from build123d import *

# Parameters (mm, degrees)
SKETCH1_W           = 30
SKETCH1_H           = 34
SKETCH1_R           = 1.625
BOSS_EXTRUDE1_DEPTH = 6
BOSS_EXTRUDE3_START = -6
SKETCH2_R           = 10
SKETCH2_R_2         = 4.05
BOSS_EXTRUDE3_DEPTH = 6
SKETCH3_R           = 2.1
BOSS_EXTRUDE4_DEPTH = 21.376405408
CUT_EXTRUDE1_START  = -10
CUT_EXTRUDE1_DEPTH  = 10
SKETCH5_W           = 4.7
SKETCH5_H           = 23.2
BOSS_EXTRUDE5_DEPTH = 17.376405408
CUT_EXTRUDE2_DEPTH  = 10
SKETCH8_R           = 2.05
CUT_EXTRUDE3_DEPTH  = 10
SKETCH9_W           = 30
SKETCH9_H           = 53.05
SKETCH9_R           = 4.05
BOSS_EXTRUDE6_DEPTH = 6
SKETCH10_R          = 2.05
CUT_EXTRUDE7_DEPTH  = 10
FILLET2_R           = 3.6
FILLET3_R           = 3.6
CHAMFER1_SIZE       = 1
CHAMFER2_SIZE       = 1


with BuildPart() as part:
    # Sketch1 → Boss-Extrude1 (new body)
    with BuildSketch(Plane.XY):
        Rectangle(SKETCH1_W, SKETCH1_H)
        with Locations((-9, 12)):
            Circle(SKETCH1_R, mode=Mode.SUBTRACT)
        with Locations((9, 12)):
            Circle(SKETCH1_R, mode=Mode.SUBTRACT)
        with Locations((-9, -12)):
            Circle(SKETCH1_R, mode=Mode.SUBTRACT)
        with Locations((9, -12)):
            Circle(SKETCH1_R, mode=Mode.SUBTRACT)
    extrude(amount=-BOSS_EXTRUDE1_DEPTH)

    # Sketch2 → Boss-Extrude3 (add)
    with BuildSketch(Plane.XY.offset(BOSS_EXTRUDE3_START)):
        Polygon((-15, -17), (15, -17), (15, -64.6), (-15, -64.6), (-27.6, -64.6), (-27.6, -41.4), (-15, -41.4), align=None)
        with Locations((0, -29)):
            Circle(SKETCH2_R, mode=Mode.SUBTRACT)
        with Locations((0, -54)):
            Circle(SKETCH2_R_2, mode=Mode.SUBTRACT)
    extrude(amount=BOSS_EXTRUDE3_DEPTH)

    # Sketch3 → Boss-Extrude4 (add)
    with BuildSketch(Plane(origin=(0, 0, -6), x_dir=(-1, 0, 0), z_dir=(0, 0, -1))):
        with BuildLine():
            Line((27.6, -61), (27.6, -45))
            ThreePointArc((27.6, -45), (26.545584412, -42.454415588), (24, -41.4))
            Line((24, -41.4), (19.7, -41.4))
            Line((19.7, -41.4), (19.7, -64.6))
            Line((19.7, -64.6), (24, -64.6))
            ThreePointArc((24, -64.6), (26.545584412, -63.545584412), (27.6, -61))
        make_face()
        with Locations(Location((24, -61, 0), (0, 0, 180))):
            Circle(SKETCH3_R, mode=Mode.SUBTRACT)
        with Locations(Location((24, -45, 0), (0, 0, 180))):
            Circle(SKETCH3_R, mode=Mode.SUBTRACT)
    extrude(amount=BOSS_EXTRUDE4_DEPTH)

    # Sketch4 → Cut-Extrude1 (cut)
    with BuildSketch(Plane(origin=(0, 0, -6), x_dir=(-1, 0, 0), z_dir=(0, 0, -1)).offset(CUT_EXTRUDE1_START)):
        with BuildLine():
            ThreePointArc((27.6, -61), (26.545584412, -63.545584412), (24, -64.6))
            Line((24, -64.6), (27.6, -64.6))
            Line((27.6, -64.6), (27.6, -61))
        make_face()
        with BuildLine():
            ThreePointArc((24, -41.4), (26.545584412, -42.454415588), (27.6, -45))
            Line((27.6, -45), (27.6, -41.4))
            Line((27.6, -41.4), (24, -41.4))
        make_face()
    extrude(amount=CUT_EXTRUDE1_DEPTH, mode=Mode.SUBTRACT)

    # Sketch5 → Boss-Extrude5 (add)
    with BuildSketch(Plane(origin=(0, 0, -6), x_dir=(-1, 0, 0), z_dir=(0, 0, -1))):
        with Locations((17.35, -53)):
            Rectangle(SKETCH5_W, SKETCH5_H)
    extrude(amount=BOSS_EXTRUDE5_DEPTH)

    # Sketch7 → Cut-Extrude2 (cut)
    with BuildSketch(Plane(origin=(0, 0, -6), x_dir=(-1, 0, 0), z_dir=(0, 0, -1))):
        with BuildLine():
            ThreePointArc((0, -64.6), (-7.495331881, -61.495331881), (-10.6, -54))
            Line((-10.6, -54), (-10.6, -43.756336497))
            ThreePointArc((-10.6, -43.756336497), (-11.098006621, -40.343327835), (-12.550498477, -37.214924709))
            ThreePointArc((-12.550498477, -37.214924709), (-14.374586553, -33.286170951), (-15, -29))
            Line((-15, -29), (-15, -64.6))
            Line((-15, -64.6), (0, -64.6))
        make_face()
    extrude(amount=-CUT_EXTRUDE2_DEPTH, mode=Mode.SUBTRACT)

    # Sketch8 → Cut-Extrude3 (cut)
    with BuildSketch(Plane(origin=(10.6, 0, 0), x_dir=(0, 0, -1), z_dir=(1, 0, 0))):
        with Locations((3, -54)):
            Circle(SKETCH8_R)
    extrude(amount=-CUT_EXTRUDE3_DEPTH, mode=Mode.SUBTRACT)

    # Sketch9 → Boss-Extrude6 (add)
    with BuildSketch(Plane.XY):
        with Locations((0, 43.525)):
            Rectangle(SKETCH9_W, SKETCH9_H)
        with Locations((0, 60)):
            Circle(SKETCH9_R, mode=Mode.SUBTRACT)
        with BuildLine():
            Line((-6.706665949, 48.593809049), (6.706665949, 48.593809049))
            ThreePointArc((6.706665949, 48.593809049), (9.567126212, 47.439316621), (10.824837954, 44.622714616))
            Line((10.824837954, 44.622714616), (9.466318981, 27.423327073))
            ThreePointArc((9.466318981, 27.423327073), (8.007195381, 24.098965988), (4.799877304, 22.397928344))
            Line((4.799877304, 22.397928344), (-4.799877304, 22.397928344))
            ThreePointArc((-4.799877304, 22.397928344), (-8.007195381, 24.098965988), (-9.466318981, 27.423327073))
            Line((-9.466318981, 27.423327073), (-10.824837954, 44.622714616))
            ThreePointArc((-10.824837954, 44.622714616), (-9.567126212, 47.439316621), (-6.706665949, 48.593809049))
        make_face(mode=Mode.SUBTRACT)
    extrude(amount=-BOSS_EXTRUDE6_DEPTH)

    # Sketch10 → Cut-Extrude7 (cut)
    with BuildSketch(Plane(origin=(0, 70.05, 0), x_dir=(1, 0, 0), z_dir=(0, 1, 0))):
        with Locations(Location((0, 3, 0), (0, 0, 270))):
            Circle(SKETCH10_R)
    extrude(amount=-CUT_EXTRUDE7_DEPTH, mode=Mode.SUBTRACT)

    # Fillet2
    fillet2_edges = [part.edges().sort_by_distance(p)[0] for p in [
        (15, 70.05, -3),
        (-15, 70.05, -3),
        (-15, -41.4, -3),
    ]]
    fillet(fillet2_edges, radius=FILLET2_R)

    # Fillet3
    fillet3_edges = [part.edges().sort_by_distance(p)[0] for p in [
        (-15, -41.4, -14.688202704),
    ]]
    fillet(fillet3_edges, radius=FILLET3_R)

    # Chamfer1
    # the kernel refuses this chamfer: 1 mm, written as the material it takes off along each edge
    with BuildSketch(Plane(origin=(0, 70.05, -3), x_dir=(0, 0, 1), z_dir=(-1, 0, 0))) as chamfer1_piece_1:
        Polygon((2.05 + CHAMFER1_SIZE, 0), (2.05, -CHAMFER1_SIZE), (2.05, 0), align=None)
    revolve(axis=Axis((0, 70.05, -3), (0, 1, 0)), mode=Mode.SUBTRACT)
    with BuildSketch(Plane(origin=(-24, -45, -27.376405408), x_dir=(1, 0, 0), z_dir=(0, 1, 0))) as chamfer1_piece_2:
        Polygon((2.1 + CHAMFER1_SIZE, 0), (2.1, -CHAMFER1_SIZE), (2.1, 0), align=None)
    revolve(axis=Axis((-24, -45, -27.376405408), (0, 0, -1)), mode=Mode.SUBTRACT)
    with BuildSketch(Plane(origin=(-24, -61, -27.376405408), x_dir=(1, 0, 0), z_dir=(0, 1, 0))) as chamfer1_piece_3:
        Polygon((2.1 + CHAMFER1_SIZE, 0), (2.1, -CHAMFER1_SIZE), (2.1, 0), align=None)
    revolve(axis=Axis((-24, -61, -27.376405408), (0, 0, -1)), mode=Mode.SUBTRACT)

    # Chamfer2
    # the kernel refuses this chamfer: 1 mm, written as the material it takes off along each edge
    with BuildSketch(Plane(origin=(0, -54, 0), x_dir=(1, 0, 0), z_dir=(0, -1, 0))) as chamfer2_piece_1:
        Polygon((4.05, -CHAMFER2_SIZE), (4.05 + CHAMFER2_SIZE, 0), (4.05, 0), align=None)
    revolve(axis=Axis((0, -54, 0), (0, 0, 1)), mode=Mode.SUBTRACT)
    with BuildSketch(Plane(origin=(0, 60, 0), x_dir=(1, 0, 0), z_dir=(0, -1, 0))) as chamfer2_piece_2:
        Polygon((4.05, -CHAMFER2_SIZE), (4.05 + CHAMFER2_SIZE, 0), (4.05, 0), align=None)
    revolve(axis=Axis((0, 60, 0), (0, 0, 1)), mode=Mode.SUBTRACT)


solid = part.part
Can you work these out from the model? Positions are in its coordinate system, mm. A direction names the side the tool comes from. Round coordinates to 2 decimals unless told otherwise and drop trailing zeros. Write each loop counter-clockwise with the first axis right and the second up, starting at its lowest first coordinate (ties: lowest second). Pieces come first, ordered by that corner, then holes. Notation, with made-up numbers: (54, 63) -> (113, 63) arc R14 ccw to (113, 75) -> close; hole circle Ø9 at (-26, 56). An arc over 180 degrees is marked (long way). Use one line per item in the form item = value. Start each with the question number.
Q1. We'd pull the mould along X, two halves only. Please class faces 1 (the face through (11.084, -40.39, -3.042)), 2 (the face through (-23.031, -43.137, -16.046)), 3 (the face through (-27.6, -53, -14)): +X half, -X half, draft (parallel to the pull), parting line (faces both ways), or undercut.
Q2. Imagine slicing it at C-C (z = -3). Count the separate pieces of the cut face and the enclosed holes in it, then the cut area to 3 significant figures.
Q3. Imagine slicing it at B-B (y = 40). Please give me the cut outline in (x, z), then the cut area to 3 significant figures.
Q4. Which directions (+Z, -Z, +X, -X, +Y, -Y) give clear straight access to the entire face, cutting with the end or side of a thin tool? Please do faces 4 (the face through (10.155, 36.143, -2.958)), 5 (the face through (-21, -41.4, -13)), 6 (the face through (7.41, -61.58, -3.04)).
Q5. If I drill on probe 1 along Y at (x, z) = (0, -3.3); probe 2 along Y at (x, z) = (-1.5, -4.5); probe 3 along X at (y, z) = (-61, -16.75), over which ranges is the centre line in solid material (lowest first)? Write a range as [from, to].
Q6. Imagine slicing it at D-D (y = 9). Please give me the cut outline in (x, z), then the cut area to 3 significant figures.
Q7. Imagine slicing it at A-A (z = -21.25). Please give me the cut outline in (x, y), then the cut area to 3 significant figures.
Q8. I'm going to push flat-ended pins straight in: P1, Ø10.5, axis at x = 0, y = -54, coming from the -Z side; P2, Ø2.5, axis at y = -54, z = -3, coming from the +X side; P3, Ø5.5, axis at x = 0, z = -3, coming from the +Y side; P4, Ø16, axis at x = 0, y = -29, coming from the -Z side. Where does each tip first touch, or does it pass through?
Worked out:
q1.face_1 = +X half
q1.face_2 = undercut
q1.face_3 = -X half
q2.separate_pieces = 1
q2.enclosed_holes = 6
q2.area = 3,160 mm^2
q3.outline = (-15, -6) -> (-10.46, -6) -> (-10.46, 0) -> (-15, 0) -> close; (10.46, -6) -> (15, -6) -> (15, 0) -> (10.46, 0) -> close
q3.area = 54.5 mm^2
q4.face_4 = +Z, -Z
q4.face_5 = +Z, -Z, -X, +Y
q4.face_6 = +Z, -Z, +X, -Y
q5.probe_1 = [-64.6, -58.05], [-49.95, -39], [-19, 22.4], [48.59, 55.95]
q5.probe_2 = [-64.6, -57.76], [-50.24, -38.89], [-19.11, 22.4], [48.59, 56.24], [63.76, 69.12]
q5.probe_3 = [-27.6, -26.1], [-21.9, -15]
q6.outline = (-15, -6) -> (15, -6) -> (15, 0) -> (-15, 0) -> close
q6.area = 180 mm^2
q7.outline = (-27.6, -61) arc R3.6 ccw to (-24, -64.6) -> (-15, -64.6) -> (-15, -45) arc R3.6 ccw to (-18.6, -41.4) -> (-24, -41.4) arc R3.6 ccw to (-27.6, -45) -> close; hole circle Ø4.2 at (-24, -61); hole circle Ø4.2 at (-24, -45)
q7.area = 256 mm^2
q8.P1 = -6
q8.P2 = -3.85
q8.P3 = 69.75
q8.P4 = through
